Can you work these out from the model? Positions are in its coordinate system, mm. A direction names the side the tool comes from. Give positions to 0.01 mm unless a question says otherwise; leave off trailing zeros. Order: outer loops, then holes, each group sorted by start corner. A loop starts at its lowest first (then second) coordinate and runs counter-clockwise, first axis right, second up. Notation, with made-up numbers: (11, 82.5) - (49, 82.5) arc R14 ccw to (49, 95.5) - close; hole circle Ø10 at (64, 29.25). An arc over 180 degrees is marked (long way). One line per question, with ' | ' between items.
Autodesk Inventor part; units mm, degrees
ref_plane "YZ Plane" through (0, 0, 0) normal (1, 0, 0) x (0, 1, 0)
ref_plane "XZ Plane" through (0, 0, 0) normal (0, 1, 0) x (-1, 0, 0)
ref_plane "XY Plane" through (0, 0, 0) normal (0, 0, 1) x (1, 0, 0)
sketch "Sketch2" plane through (0, 0, 0) normal (1, 0, 0) x (0, 1, 0)
  circle A0 centre (0, 0) radius 10
  circle A1 centre (0, 0) radius 22
  line L0 (0, 0) -> (7.0711, -7.0711)
  line L1 (0, 0) -> (10, 0) construction
  circle A2 centre (7.0711, -7.0711) radius 1.5
  line L2 (0, 0) -> (10.8294, 10.8294)
  line L3 (0, 0) -> (15.315, 0) construction
  circle A3 centre (-7.0711, 7.0711) radius 1.5
  dimension "d3" = 20
  dimension "d4" = 44
  dimension "d16" = 10
  dimension "d17" = 45
  dimension "d18" = 3
  dimension "d19" = 45
extrude "Extrusion1" add sketch "Sketch2" along normal blind 12 contours A2 A0 | A0 L0 A2 | A3 A0 | A0 A3 | A0 A2 L0 | A1
sketch "Sketch4" plane through (0, 0, 0) normal (1, 0, 0) x (0, 0, -1)
  circle A0 centre (0, 0) radius 15.75
  circle A1 centre (15.75, 0) radius 2.55
  dimension "d9" = 31.5
  dimension "d10" = 5.1
extrude "Extrusion3" cut sketch "Sketch4" along normal blind 30 contours A0 A1 | A0 A1 picked at (14.9184, -0.4924) picked at (16.4994, -0.6699)
sketch "Sketch5" plane through (12, 0, 0) normal (1, 0, 0) x (0, 0, -1)
  circle A0 centre (15.75, 0) radius 2.55
  circle A1 centre (15.75, 0) radius 4.5
  point P0 (0, 0)
  dimension "d20" = 9
extrude "Extrusion4" cut sketch "Sketch5" against normal blind 4
sketch "Sketch6" plane through (12, 0, 0) normal (1, 0, 0) x (0, 0, -1)
  line L0 (0, 0) -> (15.5563, 15.5563)
  line L1 (0, 0) -> (22, 0) construction
  dimension "d23" = 22
  dimension "d24" = 45
ref_plane "Work Plane1" through (12, 15.5563, -15.5563) normal (0, 0.7071068, -0.7071068) x (-1, 0, 0)
sketch "Sketch7" plane through (12, 15.5563, -15.5563) normal (0, 0.7071068, -0.7071068) x (-1, 0, 0)
  line L0 (0, 22) -> (0, -22)
  line L1 (0, 0) -> (12, 0)
  circle A0 centre (6, 0) radius 2.6
  dimension "d25" = 5.2
extrude "Extrusion5" cut sketch "Sketch7" against normal blind 10
ref_plane "Work Plane2" through (12, 0, 0) normal (0, 0.7071068, -0.7071068) x (-1, 0, 0)
thread "Thread1"
mirror "Mirror1" about plane through (12, 0, 0) normal (0, 0.7071068, -0.7071068) of "Extrusion5"
sketch "Sketch8" plane through (12, 0, 0) normal (1, 0, 0) x (0, 0, -1)
  line L0 (0, 0) -> (22, 0) construction
  circle A0 centre (15.75, 0) radius 2.55
  circle A1 centre (15.75, 0) radius 5
  dimension "d33" = 10
extrude "Extrusion6" cut sketch "Sketch8" against normal blind 2
chamfer "Chamfer2" distance 0.5 angle 45 1 edges at (10, 0, -11.25)
pattern_circular "Circular Pattern1" count 4 over 360 about axis through (-10, 0, 0) along (1, 0, 0) of "Extrusion3", "Extrusion4", "Extrusion6", "Chamfer2"
mirror "Mirror2" about plane through (0, 0, 0) normal (0, 0, 1) of "Extrusion5", "Mirror1"
properties part number "Pen Holder Interface V3"
(1) If we mould it in two halves opening along Y, with no side actions, what happens to faces 3 (the face through (3.9, -13.2, 0.1)), 4 (the face through (5.92, 10.15, 19.52)), 5 (the face through (0, 5, -9)), 6 (the face through (6.338, -13.893, 10.247))? For each: released by +Y, released by -Y, zero draft, split by the parting line, or undercut.
Answer below:
face 3: undercut | face 4: split by the parting line | face 5: zero draft | face 6: undercut
(2) Imagine slicing it at A-A (y = 0). Count the separate pieces of the cut face and the enclosed holes in it, and give its area (3 significant figures).
Answer below:
separate pieces: 4 | enclosed holes: 0 | area: 130 mm^2
(3) Will these pins go through, and if not, where does the flat tip stop? pin 1 (7 mm diameter, centred on y = -15.5, z = 1, fed in from +X); pin 2 (8 mm diameter, centred on y = 15.75, z = 0, fed in from +X); pin 3 (3 mm diameter, centred on x = 6.5, y = 17, fed in from +Z).
Answer below:
pin 1: x = 9.53 | pin 2: x = 8 | pin 3: z = 14.31
(4) On a 3-axis mill with a long thin cutter (end or side, diameter ignored), from which of +Z, -Z, +X, -X, +Y, -Y can I reach the whole of each face in a straight line? I mean faces 1 (the face through (8, 18, -2)), 2 (the face through (5.92, -6.93, -7.21)). Say none if no direction works.
Answer below:
face 1: +X | face 2: +X, -X
(5) If I drill on line 1 (Z direction, x = 7.5, y = 3); line 2 (Z direction, x = 6.5, y = 8.5); line 3 (X direction, y = -11, z = -12.5), over which ranges is the centre line in solid material (lowest first)?
Answer below:
line 1: -21.79 to -9.54, 9.54 to 21.79 | line 2: -20.29 to -12.11, -8.47 to -5.27, 5.27 to 8.47, 12.11 to 20.29 | line 3: 0 to 3.63, 8.37 to 12
(6) Imagine slicing it at B-B (x = 7.25). List the corners of the cut face in (y, z) for me.
Answer below:
outline: (-17.08, -13.86) - (-10.1, -6.87) - (-6.87, -10.1) - (-13.86, -17.08) arc R22 ccw to (13.86, -17.08) - (6.87, -10.1) - (10.1, -6.87) - (17.08, -13.86) arc R22 ccw to (17.08, 13.86) - (10.1, 6.87) - (6.87, 10.1) - (13.86, 17.08) arc R22 ccw to (-13.86, 17.08) - (-6.87, 10.1) - (-10.1, 6.87) - (-17.08, 13.86) arc R22 ccw to start; hole circle Ø5.1 at (-15.75, 0); hole (-8.05, 5.93) arc R10 ccw to (5.93, -8.05) arc R1.5 cw to (8.05, -5.93) arc R10 ccw to (-5.93, 8.05) arc R1.5 cw to start; hole circle Ø5.1 at (0, -15.75); hole circle Ø5.1 at (0, 15.75); hole circle Ø5.1 at (15.75, 0)
